The model under review builds one solid part; all positions refer to its coordinate system, in mm. A direction names the side the tool comes from. Round coordinates to 2 decimals unless told otherwise and drop trailing zeros. Order: outer loops, then holes, each group sorted by start corner. A loop starts at its lowest first (then second) coordinate and runs counter-clockwise, first axis right, second up. Notation, with made-up numbers: M 25.25,9.5 L 79.25,9.5 A24 cw 79.25,34.5 Z; hole C -34,-17 d1. An arc over 180 degrees is marked long. One line per item, written item: value. Start each with the question number.
from build123d import *

# Parameters (mm, degrees)
SKETCH1_R           = 7.62
BOSS_EXTRUDE1_DEPTH = 1.27
BOSS_EXTRUDE2_DEPTH = 7.62
SKETCH3_R           = 5.715
BOSS_EXTRUDE3_DEPTH = 1.27
SKETCH4_R           = 6.35
BOSS_EXTRUDE4_DEPTH = 1.27
FILLET1_R           = 0.254
SKETCH5_R           = 2.032
CUT_EXTRUDE1_DEPTH  = 11.43


with BuildPart() as part:
    # Sketch1 → Boss-Extrude1 (new body)
    with BuildSketch(Plane.XY):
        Circle(SKETCH1_R)
    extrude(amount=BOSS_EXTRUDE1_DEPTH)

    # Sketch2 → Boss-Extrude2 (add)
    with BuildSketch(Plane.XY.offset(1.27)):
        Polygon((3.666174209, 6.35), (-3.666174209, 6.35), (-7.332348419, 0), (-3.666174209, -6.35), (3.666174209, -6.35), (7.332348419, 0), align=None)
    extrude(amount=BOSS_EXTRUDE2_DEPTH)

    # Sketch3 → Boss-Extrude3 (add)
    with BuildSketch(Plane.XY.offset(8.89)):
        Circle(SKETCH3_R)
    extrude(amount=BOSS_EXTRUDE3_DEPTH)

    # Sketch4 → Boss-Extrude4 (add)
    with BuildSketch(Plane.XY.offset(10.16)):
        Circle(SKETCH4_R)
    extrude(amount=BOSS_EXTRUDE4_DEPTH)

    # Fillet1
    fillet1_edges = [part.edges().sort_by_distance(p)[0] for p in [
        (-5.715, 0, 10.16),
        (-6.35, 0, 10.16),
    ]]
    fillet(fillet1_edges, radius=FILLET1_R)

    # Sketch5 → Cut-Extrude1 (cut)
    with BuildSketch(Plane.XY.offset(11.43)):
        Circle(SKETCH5_R)
    extrude(amount=-CUT_EXTRUDE1_DEPTH, mode=Mode.SUBTRACT)


solid = part.part
Item 1: Clearance check with flat-ended pins moving along their axes: P1, Ø4.5, axis at x = 0, y = 0, coming from the -Z side; P2, Ø4, axis at x = 5, z = 8.5, coming from the +Y side; P3, Ø3.5, axis at x = 0, z = 3.5, coming from the -Y side. State where each tip first meets the part, or that it passes through.
Item 2: Consider section B-B, the plane z = 5.5. Give the boundary of the cut face in (x, y).
Item 3: The part is to be moulded in two halves that separate along Z. For faces 6 (the cylindrical face through (-1.38, -6.2, 10.91)), 7 (the flat face through (-2, 2, 11.43)), 8 (the cylindrical face through (5.45, 1.72, 9.39)), say which applies: pulls with the +Z half, pulls with the -Z half, needs draft (parallel to the pull), parting line crosses it, or undercut.
Item 4: Consider section C-C, the plane x = 6.75. Give the boundary of the cut face in (y, z), then the cut area to 3 significant figures.
Item 5: Wall thickness on L1, parallel to Y at x = 0, z = 9.25 (3 decimals); L2, parallel to Y at x = 0, z = 7.5; L3, parallel to Z at x = -3.5, y = 5: over which ranges is each line inside the solid? List them lowest first.
Item 6: Consider section A-A, the plane x = 0. Give the boundary of the cut face in (y, z) (3 decimals), then the cut area to 3 significant figures.
Item 7: Machinability: for faces 1 (the flat face through (5.525, 3.131, 5.027)), 2 (the flat face through (-5.474, 3.219, 5.027)), 3 (the flat face through (6, -3, 1.27)), 4 (the flat face through (0, 6.35, 5)), 5 (the flat face through (5.474, -3.219, 5.027)), which of the approach directions +Z, -Z, +X, -X, +Y, -Y give a long, thin tool a straight path to every point of the face, cutting with its end or side? Answer none if there is none.
Computed:
1. P1: stops at z = 0
1. P2: stops at y = 6.35
1. P3: stops at y = -6.35
2. outline: M -7.33,0 L -3.67,-6.35 L 3.67,-6.35 L 7.33,0 L 3.67,6.35 L -3.67,6.35 Z; hole C 0,0 d4.06
3. face 6: needs draft
3. face 7: pulls with the +Z half
3. face 8: undercut
4. outline: M -3.54,0 L 3.54,0 L 3.54,1.27 L 1.01,1.27 L 1.01,8.89 L -1.01,8.89 L -1.01,1.27 L -3.54,1.27 Z
4. area: 24.4 mm^2
5. L1: y = -5.715 to -2.032, 2.032 to 5.715
5. L2: y = -6.35 to -2.03, 2.03 to 6.35
5. L3: z = 0 to 8.89, 10.16 to 11.43
6. outline: M -7.62,0 L -2.032,0 L -2.032,11.43 L -6.35,11.43 L -6.35,10.414 A0.254 ccw -6.096,10.16 L -5.969,10.16 A0.254 cw -5.715,9.906 L -5.715,8.89 L -6.35,8.89 L -6.35,1.27 L -7.62,1.27 Z; M 2.032,0 L 7.62,0 L 7.62,1.27 L 6.35,1.27 L 6.35,8.89 L 5.715,8.89 L 5.715,9.906 A0.254 cw 5.969,10.16 L 6.096,10.16 A0.254 ccw 6.35,10.414 L 6.35,11.43 L 2.032,11.43 Z
6. area: 100 mm^2
7. face 1: +Z, +X, +Y
7. face 2: +Z, -X, +Y
7. face 3: +Z
7. face 4: +Z, +X, -X, +Y
7. face 5: +Z, +X, -Y
